Could you check a few things on this drawing? It's one solid part, dimensions in mm from its lowest x, y, z. Give positions to 0.01 mm unless a question says otherwise; leave off trailing zeros. Write each loop counter-clockwise with the first axis right and the second up, starting at its lowest first coordinate (ties: lowest second). Pieces come first, ordered by that corner, then holes. Notation, with made-up numbers: M 74,34 L 115,34 A10 ccw 115,39 Z; hole C 2,66 d2. An arc over 180 degrees is marked long. Answer as CSV lines item,"result". Start each with the question number.
Q1. Suppose I cut it at B-B (x = 17). Write out the boundary of the cut face in (y, z).
Q2. Suppose I cut it at D-D (x = 3.5). Write out the boundary of the cut face in (y, z).
Q3. If I drill on line 1 along Y through (x, z) = (18, 2.65); line 2 along X through (y, z) = (47.5, 3.25); line 3 along X through (y, z) = (46, 3), over which ranges is the centre line in solid material (lowest first)?
Q4. For pin 1 (1.5 mm diameter, centred on x = 22, y = 30, fed in from -Z), with a flat end and sliding along its axis, tell me the tip position at first contact or that it passes through.
Q5. Thinking about a two-plate mould opening in X: for the marked faces 1, 2, 3 and 4, which applies, +X half, -X half, draft (parallel to the pull), parting line (faces both ways), or undercut?
Q6. Suppose I cut it at C-C (y = 4). Write out the boundary of the cut face in (x, z), then the cut area to 3 significant figures.
Q7. Suppose I cut it at A-A (y = 45). Write out the boundary of the cut face in (x, z) (3 decimals).
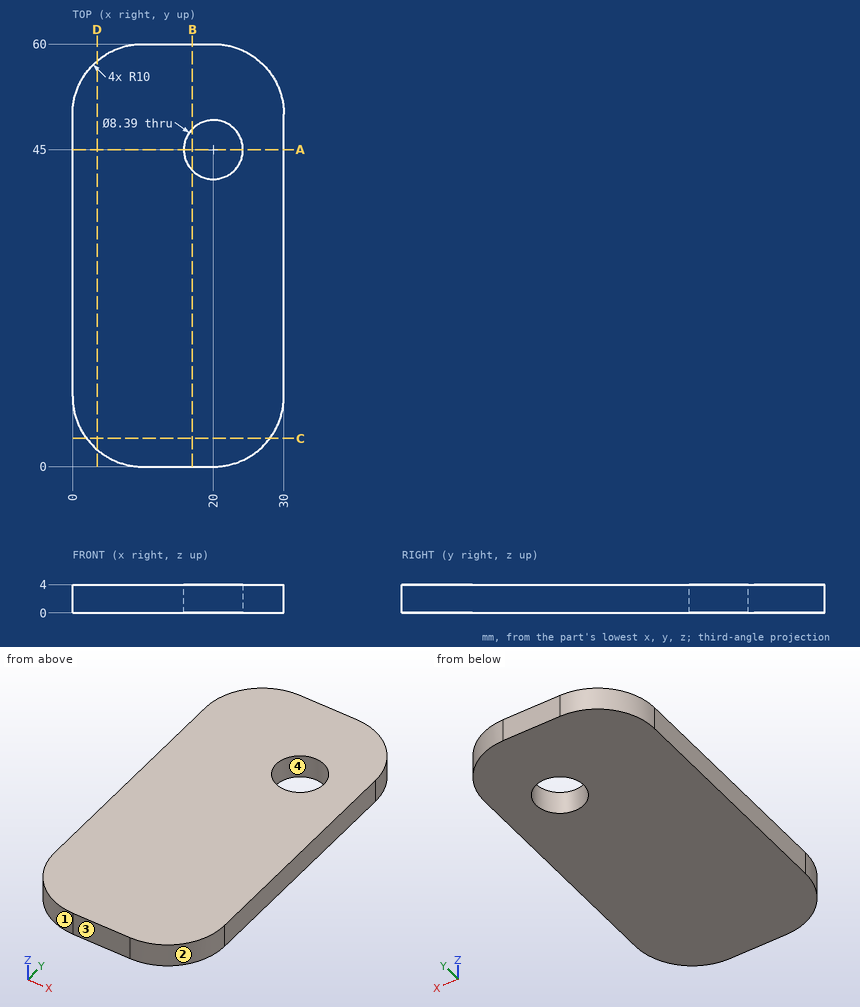
Resolved:
1,outline,"M 0,0 L 42.07,0 L 42.07,4 L 0,4 Z; M 47.93,0 L 60,0 L 60,4 L 47.93,4 Z"
2,outline,"M 2.4,0 L 57.6,0 L 57.6,4 L 2.4,4 Z"
3,line 1,"0 to 41.31, 48.69 to 60"
3,line 2,"0 to 16.63, 23.37 to 30"
3,line 3,"0 to 15.93, 24.07 to 30"
4,pin 1,"z = 0"
5,face 1,"-X half"
5,face 2,"+X half"
5,face 3,"draft"
5,face 4,"undercut"
6,outline,"M 2,0 L 28,0 L 28,4 L 2,4 Z"
6,area,"104 mm^2"
7,outline,"M 0,0 L 15.805,0 L 15.805,4 L 0,4 Z; M 24.195,0 L 30,0 L 30,4 L 24.195,4 Z"
